For this review, take the finished solid that the model builds, in its own axes (mm). Give positions to 0.01 mm unless a question says otherwise; leave off trailing zeros. Write each loop counter-clockwise with the first axis right and the second up, starting at its lowest first coordinate (ties: lowest second). Pieces come first, ordered by that corner, then holes. Notation, with made-up numbers: (24, 32.25) -> (78, 32.25) arc R14 ccw to (78, 56.25) -> close; hole circle Ø11 at (72, 44.5). An arc over 180 degrees is marked (long way). Return JSON: item names as keys, results as strings.
from build123d import *

# Parameters (mm, degrees)
SKETCH1_R            = 2.0828
BOSS_EXTRUDE1_DEPTH  = 3.175
M3_CLEARANCE_HOLE1_D = 3.2
SKETCH5_W            = 19.8
SKETCH5_H            = 4.5
CUT_EXTRUDE1_DEPTH   = 265.974627323
SKETCH7_R            = 2.413
CUT_EXTRUDE2_DEPTH   = 265.974627323
SKETCH8_R            = 3.81
CUT_EXTRUDE3_DEPTH   = 265.974627323


with BuildPart() as part:
    # Sketch1 → Boss-Extrude1 (new body)
    with BuildSketch(Plane(origin=(0, 0, 0), x_dir=(1, 0, 0), z_dir=(0, 1, 0))):
        Polygon((28.855389821, 184.15), (123.544610179, 184.15), (176.5, 131.194610179), (182.5, 125.194610179), (190.5, 117.194610179), (190.5, 22.505389821), (182.5, 14.505389821), (176.5, 8.505389821), (137.544610179, -30.45), (131.544610179, -36.45), (123.544610179, -44.45), (28.855389821, -44.45), (20.855389821, -36.45), (14.855389821, -30.45), (-24.1, 8.505389821), (-30.1, 14.505389821), (-38.1, 22.505389821), (-38.1, 117.194610179), (-30.1, 125.194610179), (-24.1, 131.194610179), align=None)
        with Locations(Location((24.384, 12.7, 0), (0, 0, 270))):
            Circle(SKETCH1_R, mode=Mode.SUBTRACT)
        with Locations(Location((128.016, 12.7, 0), (0, 0, 90))):
            Circle(SKETCH1_R, mode=Mode.SUBTRACT)
        with Locations(Location((128.016, 127, 0), (0, 0, 270))):
            Circle(SKETCH1_R, mode=Mode.SUBTRACT)
        with Locations(Location((24.384, 127, 0), (0, 0, 90))):
            Circle(SKETCH1_R, mode=Mode.SUBTRACT)
    extrude(amount=BOSS_EXTRUDE1_DEPTH)

    # M3 Clearance Hole1 (through all)
    with Locations(Plane(origin=(0, 3.175, 0), x_dir=(1, 0, 0), z_dir=(0, 1, 0))):
        with Locations((-31.5214, 106.313101446), (-31.5214, 91.073101446), (-31.5214, 55.8795536), (-31.5214, 40.6395536), (-31.5214, 25.230335162), (-16.2814, 25.230335162), (68.58, -37.8714), (83.82, -37.8714), (183.9214, 25.230335162), (168.6814, 25.230335162), (183.9214, 40.6395536), (183.9214, 55.8795536), (183.9214, 91.073101446), (183.9214, 106.313101446)):
            Hole(M3_CLEARANCE_HOLE1_D / 2)

    # Sketch5 → Cut-Extrude1 (cut, through all)
    with BuildSketch(Plane(origin=(0, 3.175, 0), x_dir=(1, 0, 0), z_dir=(0, 1, 0))):
        with Locations((76.2, 97.5)):
            Rectangle(SKETCH5_W, SKETCH5_H)
    extrude(amount=-CUT_EXTRUDE1_DEPTH, mode=Mode.SUBTRACT)

    # Sketch7 → Cut-Extrude2 (cut, through all)
    with BuildSketch(Plane(origin=(0, 3.175, 0), x_dir=(1, 0, 0), z_dir=(0, 1, 0))):
        with Locations(Location((50.8, 154.263560488, 0), (0, 0, 270))):
            Circle(SKETCH7_R)
        with Locations(Location((101.6, 154.263560488, 0), (0, 0, 90))):
            Circle(SKETCH7_R)
    extrude(amount=-CUT_EXTRUDE2_DEPTH, mode=Mode.SUBTRACT)

    # Sketch8 → Cut-Extrude3 (cut, through all)
    with BuildSketch(Plane(origin=(0, 3.175, 0), x_dir=(1, 0, 0), z_dir=(0, 1, 0))):
        with Locations(Location((76.2, 140.698010266, 0), (0, 0, 270))):
            Circle(SKETCH8_R)
    extrude(amount=-CUT_EXTRUDE3_DEPTH, mode=Mode.SUBTRACT)


solid = part.part
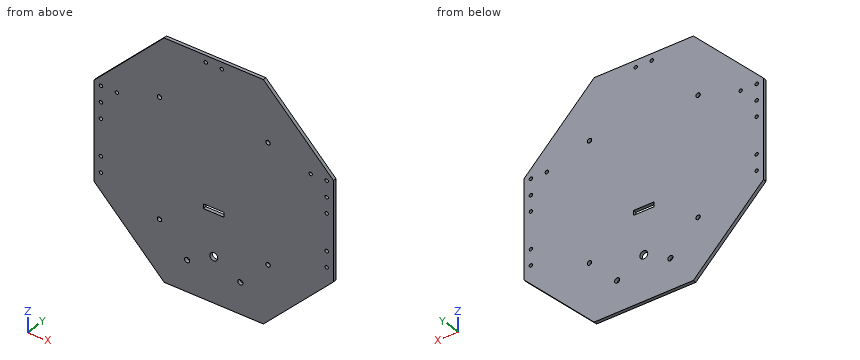
1. Add section C-C, the plane z = 11.5. State the section outline as (x, y) points (3 decimals), plus the area to 3 significant figures.
Results found:
{"outline": "(-4.095, 0) -> (156.495, 0) -> (156.495, 3.175) -> (-4.095, 3.175) -> close", "area": "510 mm²"}
2. Add section D-D, the plane z = -18.5. State the section outline as (x, y) points (3 decimals), plus the area to 3 significant figures.
Results found:
{"outline": "(-34.095, 0) -> (186.495, 0) -> (186.495, 3.175) -> (-34.095, 3.175) -> close", "area": "700 mm²"}
3. Add section B-B, the plane y = 2.1. Count the separate pieces of the cut face and the enclosed holes in it, plus the area to 3 significant figures.
Results found:
{"separate pieces": "1", "enclosed holes": "22", "area": "43,000 mm²"}
4. For pin 1 (1.5 mm diameter, centred on x = 153.5, y = 2, fed in from -Z), flat-tipped, find the tip position at first contact; note if it passes through.
Results found:
{"pin 1": "stops at z = -154.94"}
5. To check wall thickness, follow probe 1 along Z at (x, y) = (83.82, 0.9); probe 2 along X at (y, z) = (0.45, -106); probe 3 along Z at (x, y) = (72, 2.6). State the ranges of each line that lie inside material, in increasing order.
Results found:
{"probe 1": "z = -184.15 to -99.75, -95.25 to 36.27, 39.47 to 44.45", "probe 2": "x = -38.1 to -33.09, -29.95 to 182.35, 185.49 to 190.5", "probe 3": "z = -184.15 to -99.75, -95.25 to 44.45"}
6. Add section A-A, the plane x = 76.2. State the section outline as (y, z) points (3 decimals), plus the area to 3 significant figures.
Results found:
{"outline": "(0, -184.15) -> (3.175, -184.15) -> (3.175, -144.508) -> (0, -144.508) -> close; (0, -136.888) -> (3.175, -136.888) -> (3.175, -99.75) -> (0, -99.75) -> close; (0, -95.25) -> (3.175, -95.25) -> (3.175, 44.45) -> (0, 44.45) -> close", "area": "687 mm²"}
